from build123d import *

# Parameters (mm, degrees)
BOSS_EXTRUDE1_DEPTH = 19
SKETCH2_R           = 11
CUT_EXTRUDE1_DEPTH  = 19
SKETCH3_R           = 11
CUT_EXTRUDE3_DEPTH  = 422
SKETCH4_W           = 64
SKETCH4_H           = 64
BOSS_EXTRUDE2_DEPTH = 45
CUT_EXTRUDE4_DEPTH  = 51
BOSS_EXTRUDE3_DEPTH = 13


with BuildPart() as part:
    # Sketch1 → Boss-Extrude1 (new body)
    with BuildSketch(Plane(origin=(0, 0, 0), x_dir=(1, 0, 0), z_dir=(0, 1, 0))):
        with BuildLine():
            Line((-32, 114), (-32, 0))
            ThreePointArc((-32, 0), (0, -32), (32, 0))
            Line((32, 0), (32, 114))
            ThreePointArc((32, 114), (0, 146), (-32, 114))
        make_face()
    extrude(amount=BOSS_EXTRUDE1_DEPTH)

    # Sketch2 → Cut-Extrude1 (cut)
    with BuildSketch(Plane(origin=(0, 19, 0), x_dir=(1, 0, 0), z_dir=(0, 1, 0))):
        with Locations(Location((0, 0, 0), (0, 0, 270))):
            Circle(SKETCH2_R)
    extrude(amount=-CUT_EXTRUDE1_DEPTH, mode=Mode.SUBTRACT)

    # Sketch3 → Cut-Extrude3 (cut)
    with BuildSketch(Plane(origin=(0, 19, 0), x_dir=(1, 0, 0), z_dir=(0, 1, 0))):
        with Locations(Location((0, 114, 0), (0, 0, 270))):
            Circle(SKETCH3_R)
    extrude(amount=-CUT_EXTRUDE3_DEPTH, mode=Mode.SUBTRACT)

    # Sketch4 → Boss-Extrude2 (add)
    with BuildSketch(Plane(origin=(0, 19, 0), x_dir=(1, 0, 0), z_dir=(0, 1, 0))):
        with Locations((0, 57)):
            Rectangle(SKETCH4_W, SKETCH4_H)
    extrude(amount=BOSS_EXTRUDE2_DEPTH)

    # Sketch5 → Cut-Extrude4 (cut)
    with BuildSketch(Plane.XY.offset(-25)):
        Polygon((32, 64), (-19, 64), (32, 13), align=None)
    extrude(amount=-CUT_EXTRUDE4_DEPTH, mode=Mode.SUBTRACT)

    # Sketch6 → Boss-Extrude3 (add)
    with BuildSketch(Plane.XY.offset(-25)):
        Polygon((32, 13), (32, 64.70943725), (-19, 64), align=None)
    extrude(amount=-BOSS_EXTRUDE3_DEPTH)


solid = part.part
Could you check a few things on this model? Use its own coordinates, in mm. A direction names the side the tool comes from. Round coordinates to 2 decimals unless told otherwise and drop trailing zeros. Order: outer loops, then holes, each group sorted by start corner. A loop starts at its lowest first (then second) coordinate and runs counter-clockwise, first axis right, second up.
Q1. Please list where these lines run through material, in increasing order: probe 1 along Z at (x, y) = (3.5, 54); probe 2 along X at (y, z) = (5.25, -114); probe 3 along Y at (x, z) = (1.5, -138.5).
Geometry says:
probe 1: z = -89 to -76, -38 to -25
probe 2: x = -32 to -11, 11 to 32
probe 3: y = 0 to 19
Q2. I'm going to push flat-ended pins straight in: P1, Ø1.5, axis at x = -1.5, z = -91, coming from the +Y side; P2, Ø4, axis at y = 22, z = -51, coming from the +X side; P3, Ø3, axis at y = 51, z = -58.5, coming from the +X side; P4, Ø17.5, axis at x = 0, z = -114, coming from the +Y side. Where does each tip first touch, or does it pass through?
Geometry says:
P1: stops at y = 19
P2: stops at x = 25
P3: stops at x = -4.5
P4: passes through
Q3. Imagine slicing it at C-C, the plane y = 52. List the corners of the cut face in (x, z) for me, then the cut area to 3 significant figures.
Geometry says:
outline: (-32, -89) - (32, -89) - (32, -76) - (-7, -76) - (-7, -38) - (32, -38) - (32, -25) - (-32, -25) - close
area: 2,610 mm2
Q4. Imagine slicing it at B-B, the plane x = 0. List the corners of the cut face in (y, z) for me.
Geometry says:
outline: (0, -146) - (19, -146) - (19, -125) - (0, -125) - close; (0, -103) - (19, -103) - (19, -89) - (64, -89) - (64, -76) - (45, -76) - (45, -38) - (64.26, -38) - (64.26, -25) - (19, -25) - (19, -11) - (0, -11) - close; (0, 11) - (19, 11) - (19, 32) - (0, 32) - close
Q5. Which directions (+Z, -Z, +X, -X, +Y, -Y) give clear straight access to the entire face, cutting with the end or side of a thin tool? Please do faces 4 (the face through (0, 41, -89)), 5 (the face through (-0.704, 9.367, 31.992)), 6 (the face through (6, 39, -57)), 7 (the face through (-8, 19, 9)).
Geometry says:
face 4: -Z, +X, -X, +Y
face 5: +Z, +Y, -Y
face 6: +X, +Y
face 7: +Z, +X, -X, +Y
Q6. Thinking about a two-plate mould opening in X: for faces 1 (the face through (-10.74, 9.63, -2.38)), 2 (the face through (32, 10, -56)), 3 (the face through (-15, 64, -79)), which applies, released by +X, released by -X, zero draft, split by the parting line, or undercut?
Geometry says:
face 1: undercut
face 2: released by +X
face 3: zero draft
Q7. Imagine slicing it at D-D, the plane y = 4. List the corners of the cut face in (x, z) for me.
Geometry says:
outline: (-32, -114) arc R32 ccw to (32, -114) - (32, 0) arc R32 ccw to (-32, 0) - close; hole circle Ø22 at (0, -114); hole circle Ø22 at (0, 0)
Q8. Imagine slicing it at A-A, the plane y = 16. List the corners of the cut face in (x, z) for me.
Geometry says:
outline: (-32, -114) arc R32 ccw to (32, -114) - (32, -76) - (29, -76) - (29, -38) - (32, -38) - (32, 0) arc R32 ccw to (-32, 0) - close; hole circle Ø22 at (0, -114); hole circle Ø22 at (0, 0)
